Here's how the part is built. I have some questions about the finished solid (model axes, mm). A direction names the side the tool comes from. Round coordinates to 2 decimals unless told otherwise and drop trailing zeros. Loops run counter-clockwise (first coordinate to the right, second up) from the corner with the lowest first, then second, coordinate; pieces in that order, holes last. Notation, with made-up numbers: M 25,-17 L 73,-17 A26 cw 73,8 Z; hole C 34,1 d8. An arc over 180 degrees is marked long. Answer as a JSON object with one key per item and string values.
from build123d import *

# Parameters (mm, degrees)
SKETCH_1_W          = 15
SKETCH_1_H          = 15
SKETCH_1_W_2        = 12
SKETCH_1_H_2        = 12
EXTRUDE_1_DEPTH     = 140
SKETCH_3_R          = 4
CUT_EXTRUDE_1_DEPTH = 22
SKETCH_4_R          = 2
CUT_EXTRUDE_2_DEPTH = 75
SKETCH_5_R          = 2
CUT_EXTRUDE_3_DEPTH = 24
SKETCH_6_R          = 2.5
CUT_EXTRUDE_4_DEPTH = 142.000886522
SKETCH_7_R          = 2.5
CUT_EXTRUDE_5_DEPTH = 142.000886522


with BuildPart() as part:
    # 草图1 → 凸台-拉伸1 (new body)
    with BuildSketch(Plane.XY):
        Rectangle(SKETCH_1_W, SKETCH_1_H)
        Rectangle(SKETCH_1_W_2, SKETCH_1_H_2, mode=Mode.SUBTRACT)
    extrude(amount=EXTRUDE_1_DEPTH)

    # 草图3 → 切除-拉伸1 (cut)
    with BuildSketch(Plane(origin=(0, 7.5, 0), x_dir=(1, 0, 0), z_dir=(0, 1, 0))):
        with Locations(Location((0, -30, 0), (0, 0, 270))):
            Circle(SKETCH_3_R)
    extrude(amount=-CUT_EXTRUDE_1_DEPTH, mode=Mode.SUBTRACT)

    # 草图4 → 切除-拉伸2 (cut)
    with BuildSketch(Plane.XZ.offset(7.5)):
        with Locations(Location((0, 130, 0), (0, 0, 270))):
            Circle(SKETCH_4_R)
        with Locations(Location((0, 115, 0), (0, 0, 270))):
            Circle(SKETCH_4_R)
    extrude(amount=-CUT_EXTRUDE_2_DEPTH, mode=Mode.SUBTRACT)

    # 草图5 → 切除-拉伸3 (cut)
    with BuildSketch(Plane(origin=(7.5, 0, 0), x_dir=(0, 0, -1), z_dir=(1, 0, 0))):
        with Locations((-105, 0)):
            Circle(SKETCH_5_R)
        with Locations((-75, 0)):
            Circle(SKETCH_5_R)
    extrude(amount=-CUT_EXTRUDE_3_DEPTH, mode=Mode.SUBTRACT)

    # 草图6 → 切除-拉伸4 (cut, through all)
    with BuildSketch(Plane.XZ.offset(7.5)):
        with Locations(Location((0, 50, 0), (0, 0, 270))):
            Circle(SKETCH_6_R)
        with Locations(Location((0, 10, 0), (0, 0, 90))):
            Circle(SKETCH_6_R)
    extrude(amount=-CUT_EXTRUDE_4_DEPTH, mode=Mode.SUBTRACT)

    # 草图7 → 切除-拉伸5 (cut, through all)
    with BuildSketch(Plane(origin=(0, 7.5, 0), x_dir=(1, 0, 0), z_dir=(0, 1, 0))):
        with Locations(Location((0, -90, 0), (0, 0, 270))):
            Circle(SKETCH_7_R)
    extrude(amount=-CUT_EXTRUDE_5_DEPTH, mode=Mode.SUBTRACT)


solid = part.part
Item 1: If I drill on L1, parallel to Y at x = 1.5, z = 82.5; L2, parallel to X at y = 6.65, z = 50; L3, parallel to Y at x = 6.35, z = 75, over which ranges is the centre line in solid material (lowest first)? Write a range as from..to.
Solution:
{"L1": "y = -7.5..-6, 6..7.5", "L2": "x = -7.5..-2.5, 2.5..7.5", "L3": "y = -7.5..-2, 2..7.5"}
Item 2: We'd pull the mould along Z, two halves only. Please class faces 1 (the face through (6.76, 0.601, 73.092)), 2 (the face through (-6, 0, 69)), 3 (the face through (6.76, 0.601, 103.092)): +Z half, -Z half, draft (parallel to the pull), parting line (faces both ways), or undercut.
Solution:
{"face 1": "undercut", "face 2": "draft", "face 3": "undercut"}
Item 3: For P1, Ø3.5, axis at x = 0, z = 115, coming from the +Y side; P2, Ø5, axis at x = 0, z = 130, coming from the +Y side, each with a flat end and sliding along its axis, tell me the tip position at first contact or that it passes through.
Solution:
{"P1": "passes through", "P2": "stops at y = 7.5"}
Item 4: I want a section at B-B on z = 130. List the corners of the cut face in (x, y) for me, plus the area to 3 significant figures.
Solution:
{"outline": "M -7.5,-7.5 L -2,-7.5 L -2,-6 L -6,-6 L -6,6 L -2,6 L -2,7.5 L -7.5,7.5 Z; M 2,-7.5 L 7.5,-7.5 L 7.5,7.5 L 2,7.5 L 2,6 L 6,6 L 6,-6 L 2,-6 Z", "area": "69.0 mm2"}
Item 5: For faces 4 (the face through (6, 0, 69)), 5 (the face through (-6.74, 0.601, 103.092)), which set-ups out of +Z, -Z, +X, -X, +Y, -Y let a thin tool reach every point of the face, with its end or its side?
Solution:
{"face 4": "+Z, -Z", "face 5": "+X, -X"}
Item 6: I want a section at C-C on z = 109.5. List the corners of the cut face in (x, y) for me, plus the area to 3 significant figures.
Solution:
{"outline": "M -7.5,-7.5 L 7.5,-7.5 L 7.5,7.5 L -7.5,7.5 Z; hole M -6,-6 L 6,-6 L 6,6 L -6,6 Z", "area": "81.0 mm2"}
Item 7: I want a section at A-A on y = 4.5. List the corners of the cut face in (x, z) for me.
Solution:
{"outline": "M -7.5,0 L -6,0 L -6,140 L -7.5,140 Z; M 6,0 L 7.5,0 L 7.5,140 L 6,140 Z"}
Item 8: I want a section at D-D on z = 31.5. List the corners of the cut face in (x, y) for me.
Solution:
{"outline": "M -7.5,-7.5 L -3.71,-7.5 L -3.71,-6 L -6,-6 L -6,6 L -3.71,6 L -3.71,7.5 L -7.5,7.5 Z; M 3.71,-7.5 L 7.5,-7.5 L 7.5,7.5 L 3.71,7.5 L 3.71,6 L 6,6 L 6,-6 L 3.71,-6 Z"}
